Geometry check sheet. Reference: the model listing, model coordinates, mm. A direction names the side the tool comes from. Give positions to 0.01 mm unless a question says otherwise; leave off trailing zeros. Loops run counter-clockwise (first coordinate to the right, second up) from the corner with the lowest first, then second, coordinate; pieces in that order, holes last. Notation, with made-up numbers: (45.5, -25) -> (101.5, -25) arc R35 cw to (101.5, 8) -> close; hole circle Ø6 at (48.5, 55.5). An arc over 180 degrees is marked (long way). Answer in a Markdown table with one row per item. Add a question column.
Autodesk Inventor part; units mm, degrees
ref_plane "YZ Plane" through (0, 0, 0) normal (1, 0, 0) x (0, 1, 0)
ref_plane "XZ Plane" through (0, 0, 0) normal (0, 1, 0) x (-1, 0, 0)
ref_plane "XY Plane" through (0, 0, 0) normal (0, 0, 1) x (1, 0, 0)
sketch "Sketch_1" plane through (0, 0, 0) normal (0, 0, 1) x (1, 0, 0)
  line L0 (5, 0) -> (-7.8, 0)
  line L1 (-7.8, 0) -> (-7.8, 5)
  line L2 (-7.8, 5) -> (-5, 5)
  line L3 (-5, 5) -> (-5, 3)
  line L4 (-5, 3) -> (0, 3)
  line L5 (0, 3) -> (0, 2)
  line L6 (0, 2) -> (4.5705, 2)
  line L7 (4.5705, 2) -> (5, 1.5705)
  line L8 (5, 1.5705) -> (5, 0)
  line L9 (5, 0) -> (-7.8, 0)
revolve "Revolution1" add sketch "Sketch_1" angle 360 about axis through (5, 0, 0) along (1, 0, 0)
thread "Thread1"
sketch "Sketch_2" plane through (-7.8, 0, 0) normal (-1, 0, 0) x (0, 1, 0)
  line L0 (-1.4434, 0) -> (-0.7217, -1.25)
  line L1 (-0.7217, -1.25) -> (0.7217, -1.25)
  line L2 (0.7217, -1.25) -> (1.4434, 0)
  line L3 (1.4434, 0) -> (0.7217, 1.25)
  line L4 (0.7217, 1.25) -> (-0.7217, 1.25)
  line L5 (-0.7217, 1.25) -> (-1.4434, 0)
extrude "Extrusion1" cut sketch "Sketch_2" against normal blind 2.5
sketch "Sketch_3" plane through (0, 0, 0) normal (0, 0, 1) x (1, 0, 0)
  line L0 (-4.5783, 0) -> (-5.3, 0)
  line L1 (-5.3, 0) -> (-5.3, 1.25)
  line L2 (-5.3, 1.25) -> (-4.5783, 0)
  line L3 (-4.5783, 0) -> (-5.3, 0)
revolve "Revolution2" cut sketch "Sketch_3" angle 360 about axis through (-4.5783, 0, 0) along (1, 0, 0)
properties part number "DBS4-5-5"
1. Gauge pin test, flat ends, axial feed: pin 1 Ø1.5 at (x, z) = (1.5, 1.5) entering from +Y; pin 2 Ø3 at (x, y) = (0, -3.5) entering from +Z; pin 3 Ø2 at (x, z) = (-3.5, 3) entering from +Y. Record the tip position at first contact, or that the pin passes through.
2. Release check for a two-part mould opening along Y. For faces 4 (the face through (-4.704, -0.047, 0.212)), 5 (the face through (-5, 3.3, 0.1)), 6 (the face through (2, 0, -2)) record: released by +Y, released by -Y, zero draft, split by the parting line, or undercut.
3. Access from +Z, -Z, +X, -X, +Y, -Y to the whole of each face (thin tool, end or side, straight path). Record for faces 1 (the face through (-6.38, -1.08, -4.88)), 2 (the face through (0, 1, -2)), 3 (the face through (-6.568, -1.088, 0.616)).
4. Sectioned sample at A-A (x = -6.5). Enter the section's corners in (y, z), plus the area to 3 significant figures.
5. Sectioned sample at C-C (x = -4). Enter the section's corners in (y, z).
6. Sectioned sample at B-B (z = 2.25). Enter the section's corners in (x, y), plus the area to 3 significant figures.
7. Sectioned sample at D-D (y = 3.5). Enter the section's corners in (x, z), plus the area to 3 significant figures.
8. Material ranges on L1, parallel to Z at x = -7.25, y = 0; L2, parallel to X at y = 3, z = -1; L3, parallel to X at y = -1.25, z = -0.25, recorded low to high. Write a range as from..to.
Response:
| question | item | result |
|---|---|---|
| 1 | pin 1 | stops at y = 1.85 |
| 1 | pin 2 | stops at z = 2.24 |
| 1 | pin 3 | stops at y = 2.24 |
| 2 | face 4 | undercut |
| 2 | face 5 | zero draft |
| 2 | face 6 | split by the parting line |
| 3 | face 1 | +X, -X |
| 3 | face 2 | +X |
| 3 | face 3 | -X |
| 4 | outline | circle Ø10 at (0, 0); hole (-1.44, 0) -> (-0.72, -1.25) -> (0.72, -1.25) -> (1.44, 0) -> (0.72, 1.25) -> (-0.72, 1.25) -> close |
| 4 | area | 73.1 mm2 |
| 5 | outline | circle Ø6 at (0, 0) |
| 6 | outline | (-7.8, -4.47) -> (-5, -4.47) -> (-5, -1.98) -> (0, -1.98) -> (0, 1.98) -> (-5, 1.98) -> (-5, 4.47) -> (-7.8, 4.47) -> close |
| 6 | area | 44.8 mm2 |
| 7 | outline | (-7.8, -3.57) -> (-5, -3.57) -> (-5, 3.57) -> (-7.8, 3.57) -> close |
| 7 | area | 20.0 mm2 |
| 8 | L1 | z = -5..-1.25, 1.25..5 |
| 8 | L2 | x = -7.8..-5 |
| 8 | L3 | x = -5.3..5 |
